Check sheet for the modelled part. Datum: model origin and axes. Units: mm. A direction names the side the tool comes from. Give positions to 0.01 mm unless a question says otherwise; leave off trailing zeros. Write each loop counter-clockwise with the first axis right and the second up, starting at its lowest first coordinate (ties: lowest second). Pieces come first, ordered by that corner, then holes. Notation, with made-up numbers: M 58,68 L 66,68 A26 cw 66,88 Z; hole C -21.75,84.5 d10. An arc over 180 degrees is marked long. Write item = value, one per line. Start each with the question number.
1) Scan lines: L1, parallel to X at y = 0.75, z = -7; L2, parallel to Y at x = 8.5, z = -3; L3, parallel to Z at x = -8.5, y = 0.45. Record each from-to range of solid material in increasing order.
2) Sectioned sample at C-C, the plane z = 3. Record the cut outline in (x, y), then the cut area to 3 significant figures.
3) Sectioned sample at D-D, the plane x = 6. Record the cut outline in (y, z), then the cut area to 3 significant figures.
4) Sectioned sample at B-B, the plane x = -1. Record the cut outline in (y, z), then the cut area to 3 significant figures.
5) Gauge pin test, flat ends, axial feed: pin 1 (0.8 mm diameter, centred on x = 8.5, y = 0.5, fed in from -Z); pin 2 (1.5 mm diameter, centred on x = -2, z = 4, fed in from +Y); pin 3 (6 mm diameter, centred on x = -6.5, z = -1.5, fed in from -Y). Record the tip position at first contact, or that the pin passes through.
6) Draft check along Z on faces 4 (the face through (5, 1, -8)), 5 (the face through (-7.5, 0.5, -4.86)), 6 (the face through (-0.1, 0.5, 8.5)), 7 (the face through (0.07, 1.591, -9.724)). Enter one of: pulls with the +Z half, pulls with the -Z half, needs draft (parallel to the pull), parting line crosses it, or undercut.
7) Set-up check for faces 1 (the face through (-5, 1, -8)), 2 (the face through (7.5, 0.5, -4.86)), 3 (the face through (0, 0, 0)): record each of +Z, -Z, +X, -X, +Y, -Y from which the full face is reachable in a straight line by a thin tool's end or side.
8) Sectioned sample at A-A, the plane y = 1.35. Record the cut outline in (x, z), then the cut area to 3 significant figures.
from build123d import *

# Parameters (mm, degrees)
SKETCH1_W           = 20
SKETCH1_H           = 17
BOSS_EXTRUDE1_DEPTH = 1
SKETCH2_R           = 1.6
SKETCH2_R_2         = 1
BOSS_EXTRUDE2_DEPTH = 20
FILLET1_R           = 10
FILLET2_R           = 0.5
SKETCH4_W           = 10
SKETCH4_H           = 12
CUT_EXTRUDE3_DEPTH  = 15.86420015


with BuildPart() as part:
    # Sketch1 → Boss-Extrude1 (new body)
    with BuildSketch(Plane(origin=(0, 0, 0), x_dir=(1, 0, 0), z_dir=(0, 1, 0))):
        Rectangle(SKETCH1_W, SKETCH1_H)
    extrude(amount=BOSS_EXTRUDE1_DEPTH)

    # Sketch2 → Boss-Extrude2 (add)
    with BuildSketch(Plane(origin=(10, 0, 0), x_dir=(0, 0, -1), z_dir=(1, 0, 0))):
        with Locations((8.800384095, 1.974416987)):
            Circle(SKETCH2_R)
        with Locations((8.800384095, 1.974416987)):
            Circle(SKETCH2_R_2, mode=Mode.SUBTRACT)
    extrude(amount=-BOSS_EXTRUDE2_DEPTH)

    # Fillet1
    # the kernel refuses this fillet: 10 mm, written as the material it adds along each edge
    with BuildSketch(Plane(origin=(-10, 0.402866989, -8.5), x_dir=(0, -1, 0), z_dir=(1, 0, 0))) as fillet1_piece_1:
        with BuildLine():
            CenterArc((8.937605274, 5.21135706), FILLET1_R, 205.046884286, 6.361578996)
            Line((-0.12201134, 0.977759676), (-0.303203672, 0.893087728))
            ThreePointArc((-0.303203672, 0.893087728), (-0.18232452, 0.473740867), (-0.19644375, 0.037548012))
            Line((-0.19644375, 0.037548012), (0, -0.2))
            ThreePointArc((0, -0.2), (0.201433495, -0.2), (0.232172223, -0.104227141))
            Line((0.232172223, -0.104227141), (0.402866989, 0))
        make_face()
    extrude(amount=20)

    # Fillet2
    fillet2_edges = [part.edges().sort_by_distance(p)[0] for p in [
        (0, 0, -8.5),
    ]]
    fillet(fillet2_edges, radius=FILLET2_R)

    # Sketch4 → Cut-Extrude3 (cut, through all)
    with BuildSketch(Plane(origin=(0, 0, 0), x_dir=(1, 0, 0), z_dir=(0, 1, 0))):
        with Locations((10, 10.859859008)):
            Rectangle(SKETCH4_W, SKETCH4_H)
        with Locations((-10, 10.859859008)):
            Rectangle(SKETCH4_W, SKETCH4_H)
    extrude(amount=CUT_EXTRUDE3_DEPTH, mode=Mode.SUBTRACT)


solid = part.part
Data:
q1.L1 = -5 to 5
q1.L2 = 0 to 1
q1.L3 = -4.86 to 8.5
q2.outline = M -10,0 L 10,0 L 10,1 L -10,1 Z
q2.area = 20.0 mm2
q3.outline = M 0,-4.86 L 1,-4.86 L 1,8.5 L 0,8.5 Z
q3.area = 13.4 mm2
q4.outline = M 0,-8.36 A0.5 ccw 0.07,-8.62 A10 cw 0.52,-9.48 A1.6 ccw long 1,-7.53 L 1,8.5 L 0,8.5 Z; hole C 1.97,-8.8 d2
q4.area = 21.7 mm2
q5.pin_1 = -4.86
q5.pin_2 = 1
q5.pin_3 = 0
q6.face_4 = needs draft
q6.face_5 = pulls with the -Z half
q6.face_6 = pulls with the +Z half
q6.face_7 = undercut
q7.face_1 = -Z, -X, +Y, -Y
q7.face_2 = -Z, +X, +Y, -Y
q7.face_3 = +Z, -Z, +X, -X, -Y
q8.outline = M -5,-10.27 L 5,-10.27 L 5,-9.58 L -5,-9.58 Z; M -5,-8.02 L 5,-8.02 L 5,-7.33 L -5,-7.33 Z
q8.area = 13.8 mm2
